Autodesk Inventor part; units mm, degrees
ref_plane "YZ Plane" through (0, 0, 0) normal (1, 0, 0) x (0, 1, 0)
ref_plane "XZ Plane" through (0, 0, 0) normal (0, 1, 0) x (-1, 0, 0)
ref_plane "XY Plane" through (0, 0, 0) normal (0, 0, 1) x (1, 0, 0)
ref_plane "Work Plane1" through (12.8382, -4.6513, 0) normal (0, 0, 1) x (1, 0, 0)
sketch "Sketch1" plane through (12.8382, -4.6513, 0) normal (0, 0, 1) x (1, 0, 0)
  circle A0 centre (-91.5002, -74.0108) radius 6
  circle A1 centre (-26.3324, -8.8429) radius 6
  ellipse E0 centre (-91.5002, -74.0108) end of major axis (-87.52, -70.0305) minor radius 5.6 (-97.1147, -74.0397) -> (-91.5291, -79.6253) ccw
  line L0 (-67.9442, -79.6253) -> (-91.5291, -79.6253)
  line L1 (-67.9442, -79.6253) -> (-49.8884, -79.6253)
  line L2 (-26.3034, -79.6253) -> (-49.8884, -79.6253)
  ellipse E1 centre (-26.3324, -74.0108) end of major axis (-22.3521, -77.991) minor radius 5.6 (-26.3034, -79.6253) -> (-20.7179, -74.0397) ccw
  line L3 (-20.7179, -8.814) -> (-20.7179, -74.0397)
  ellipse E2 centre (-26.3324, -8.8429) end of major axis (-22.3521, -4.8627) minor radius 5.6 (-20.7179, -8.814) -> (-26.3034, -3.2284) ccw
  line L4 (-91.5291, -3.2284) -> (-26.3034, -3.2284)
  ellipse E3 centre (-91.5002, -8.8429) end of major axis (-87.52, -12.8231) minor radius 5.6 (-91.5291, -3.2284) -> (-97.1147, -8.814) ccw
  line L5 (-97.1147, -74.0397) -> (-97.1147, -8.814)
  line L6 (-79.4163, -63.9268) -> (-38.4163, -63.9268)
  line L7 (-36.4163, -61.9268) -> (-36.4163, -20.9268)
  line L8 (-38.4163, -18.9268) -> (-79.4163, -18.9268)
  line L9 (-81.4163, -20.9268) -> (-81.4163, -61.9268)
  line L10 (-58.9163, -79.6253) -> (-58.9163, -3.2284)
  line L11 (-97.1147, -41.4268) -> (-20.7179, -41.4268)
  arc A2 (-81.4163, -61.9268) -> (-79.4163, -63.9268) centre (-79.4163, -61.9268) ccw
  arc A3 (-38.4163, -63.9268) -> (-36.4163, -61.9268) centre (-38.4163, -61.9268) ccw
  arc A4 (-36.4163, -20.9268) -> (-38.4163, -18.9268) centre (-38.4163, -20.9268) ccw
  arc A5 (-79.4163, -18.9268) -> (-81.4163, -20.9268) centre (-79.4163, -20.9268) ccw
  line L12 (-87.2576, -78.2534) -> (-22.0897, -13.0855)
  line L13 (-95.7429, -69.7681) -> (-30.575, -4.6003)
  point P0 (-12.8382, 4.6513)
  point P1 (-81.4163, -63.9268)
  point P2 (-36.4163, -18.9268)
  point P3 (-36.4163, -63.9268)
  point P4 (-72.931, -63.9268)
  point P5 (-36.4163, -27.4121)
  point P6 (-44.9016, -18.9268)
  point P7 (-81.4163, -55.4416)
  point P8 (-29.8782, -23.5781)
  point P9 (-75.1162, -63.9268)
  dimension "d0" = 12
  dimension "d1" = 12
  dimension "d2" = 45
  dimension "d3" = 45
  dimension "d4" = 2
extrude "Extrusion1" add sketch "Sketch1" along normal blind 18 contours A0 L0 E0 L5 | A0 L13 L9 A2 L6 L12 | L5 E0 L0 A0 | L13 L11 L10 L12 L6 A2 L9 | L9 L11 L13 | L12 L10 L6 | L9 A5 L8 L10 L13 L11 | L13 L10 L11 | L10 L12 L11 L7 A3 L6 | L10 L11 L12 | L10 L13 L8 A4 L7 L12 L11 | L10 L8 L13 | L12 L7 L11 | L13 A1 L12 L7 A4 L8 | A1 L4 E2 L3 | A1 L3 E2 L4
sketch "Sketch2" plane through (12.8382, -4.6513, 18) normal (0, 0, 1) x (1, 0, 0)
  line L0 (-44.9016, -18.9268) -> (-79.4163, -18.9268)
  arc A0 (-79.4163, -18.9268) -> (-81.4163, -20.9268) centre (-79.4163, -20.9268) ccw
  line L1 (-81.4163, -20.9268) -> (-81.4163, -55.4416)
  line L2 (-36.4163, -61.9268) -> (-36.4163, -27.4121)
  arc A1 (-38.4163, -63.9268) -> (-36.4163, -61.9268) centre (-38.4163, -61.9268) ccw
  line L3 (-72.931, -63.9268) -> (-38.4163, -63.9268)
  line L4 (-62.1589, -18.9268) -> (-55.6737, -63.9268)
  line L5 (-36.4163, -44.6695) -> (-81.4163, -38.1842)
  line L6 (-44.9016, -18.9268) -> (-79.4163, -18.9268)
  line L7 (-81.4163, -20.9268) -> (-81.4163, -55.4416)
  arc A2 (-79.4163, -18.9268) -> (-81.4163, -20.9268) centre (-79.4163, -20.9268) ccw
  line L8 (-81.4163, -27.4121) -> (-81.4163, -61.9268)
  arc A3 (-81.4163, -61.9268) -> (-79.4163, -63.9268) centre (-79.4163, -61.9268) ccw
  line L9 (-79.4163, -63.9268) -> (-44.9016, -63.9268)
  line L10 (-72.931, -63.9268) -> (-38.4163, -63.9268)
  arc A4 (-38.4163, -63.9268) -> (-36.4163, -61.9268) centre (-38.4163, -61.9268) ccw
  line L11 (-36.4163, -61.9268) -> (-36.4163, -27.4121)
  line L12 (-36.4163, -55.4416) -> (-36.4163, -20.9268)
  arc A5 (-36.4163, -20.9268) -> (-38.4163, -18.9268) centre (-38.4163, -20.9268) ccw
  line L13 (-38.4163, -18.9268) -> (-72.931, -18.9268)
  line L14 (-81.4163, -55.4416) -> (-100.4764, -69.4227)
  line L15 (-100.4764, -69.4227) -> (-100.4764, -80.6902)
  line L16 (-100.4764, -80.6902) -> (-89.2076, -83.945)
  line L17 (-89.2076, -83.945) -> (-75.1931, -71.7586)
  line L18 (-75.1931, -71.7586) -> (-72.931, -63.9268)
  line L19 (-44.9016, -18.9268) -> (-41.3617, -6.671)
  line L20 (-41.3617, -6.671) -> (-27.2892, 1.0126)
  line L21 (-27.2892, 1.0126) -> (-19.5179, 0.2355)
  line L22 (-19.5179, 0.2355) -> (-4.3296, -12.1655)
  line L23 (-4.3296, -12.1655) -> (-5.4222, -23.0912)
  line L24 (-5.4222, -23.0912) -> (-36.4163, -27.4121)
  point P0 (-12.8382, 4.6513)
  point P1 (-58.9163, -41.4268)
  point P2 (-81.4163, -55.4416)
  point P3 (-72.931, -63.9268)
  point P4 (-36.4163, -27.4121)
  point P5 (-43.7192, -14.8334)
  point P6 (-32.0634, -23.5781)
  point P7 (-25.5781, -68.5781)
  point P8 (-23.5781, -32.0634)
  point P9 (-32.0634, -23.5781)
  point P10 (-38.4163, -63.9268)
  dimension "d9" = 360
extrude "Extrusion2" cut sketch "Sketch2" against normal blind 8 contours L19 L20 L21 L22 L23 L24 L12 A5 L13 | L18 L17 L16 L15 L14 L8 A3 L9
fillet "Fillet1" radius 8 6 edges at (-28.8207, -23.5781, 10) (-23.5781, -28.8207, 10) (-24.1639, -24.1639, 10) (-63.3355, -68.5781, 10) (-68.5781, -63.3355, 10) (-67.9923, -67.9923, 10)
equation "\"d1\" = d0"
properties part number "base" material "ABS Plastic"
Geometry: final body of the model. Coordinates: model frame, mm. A direction names the side the tool comes from. Give positions to 0.01 mm unless a question says otherwise; leave off trailing zeros. Order: outer loops, then holes, each group sorted by start corner. A loop starts at its lowest first (then second) coordinate and runs counter-clockwise, first axis right, second up. Notation, with made-up numbers: (72.5, 12) -> (110.5, 12) arc R27 ccw to (110.5, 33) -> close; hole circle Ø7 at (66.25, 73). An arc over 180 degrees is marked (long way). Put each result on its own line as item: value.
Q1. Section D-D, the plane z = 5.75. Return loops of the section in (x, y), then the cut area to 3 significant figures.
Here are the results:
outline: (-82.9, -74.42) arc R6 ccw to (-74.42, -82.9) -> (-60.09, -68.58) -> (-25.58, -68.58) arc R2 ccw to (-23.58, -66.58) -> (-23.58, -32.06) -> (-9.25, -17.74) arc R6 ccw to (-17.74, -9.25) -> (-32.06, -23.58) -> (-66.58, -23.58) arc R2 ccw to (-68.58, -25.58) -> (-68.58, -60.09) -> close
area: 2,550 mm^2
Q2. Section C-C, the plane x = -62. Return loops of the section in (y, z), then the cut area to 3 significant figures.
Here are the results:
outline: (-70.49, 0) -> (-23.58, 0) -> (-23.58, 18) -> (-68.58, 18) arc R8 cw to (-70.49, 12.82) -> close
area: 838 mm^2
Q3. Material intervals for L1, parallel to X at y = -60, z = 1.25; L2, parallel to Y at x = -31, z = 7.25, sorted ascending.
Here are the results:
L1: x = -68.58 to -23.58
L2: y = -68.58 to -22.51
Q4. Reachability of faces 1 (the face through (-78, -78, 10)), 2 (the face through (-68.578, -43, 9)), 3 (the face through (-14, -14, 10)) from +Z, -Z, +X, -X, +Y, -Y: full face, straight path, thin tool, end or side. Return the list, or none.
Here are the results:
face 1: +Z, -X, -Y
face 2: +Z, -Z, -X, +Y
face 3: +Z, +X, +Y
Q5. Section B-B, the plane y = -27. Return loops of the section in (x, z), then the cut area to 3 significant figures.
Here are the results:
outline: (-68.58, 0) -> (-18.51, 0) -> (-18.51, 10.56) arc R8 cw to (-23.58, 18) -> (-68.58, 18) -> close
area: 874 mm^2
Q6. Section A-A, the plane z = 11.75. Return loops of the section in (x, y), then the cut area to 3 significant figures.
Here are the results:
outline: (-71.58, -66.58) arc R5.01 ccw to (-66.58, -71.58) -> (-63.1, -71.58) -> (-60.09, -68.58) -> (-25.58, -68.58) arc R2 ccw to (-23.58, -66.58) -> (-23.58, -32.06) -> (-20.57, -29.06) -> (-20.57, -25.58) arc R5.01 ccw to (-25.58, -20.57) -> (-29.06, -20.57) -> (-32.06, -23.58) -> (-66.58, -23.58) arc R2 ccw to (-68.58, -25.58) -> (-68.58, -60.09) -> (-71.58, -63.1) -> close
area: 2,110 mm^2
Q7. Pin query (flat end, axial travel): pin 1 (6 mm diameter, centred on x = -21.5, z = 14.5, fed in from +Y); pin 2 (5.5 mm diameter, centred on x = -36.5, z = 12, fed in from -Y); pin 3 (3 mm diameter, centred on x = -30.5, z = 8, fed in from +Y); pin 4 (5 mm diameter, centred on y = -73.5, z = 13.5, fed in from -X). Return the tip coordinate at first contact, or that it passes through.
Here are the results:
pin 1: stops at y = -21.48
pin 2: stops at y = -68.58
pin 3: stops at y = -20.51
pin 4: passes through
